Geometry: final body of the model. Coordinates: model frame, mm. Face numbers are marked on the shaded views. A direction names the side the tool comes from. Give positions to 0.01 mm unless a question says otherwise; leave off trailing zeros. Order: outer loops, then holes, each group sorted by start corner. A loop starts at its lowest first (then second) coordinate and runs counter-clockwise, first axis right, second up. Notation, with made-up numbers: (28.5, 59.25) -> (85.5, 59.25) arc R19 cw to (85.5, 85.25) -> close; hole circle Ø11 at (-16, 14.5). An arc over 180 degrees is marked (long way). Answer in a Markdown table with one row per item. Add a question column.
Q1. Set-up query: the marked faces 1 and 2. Return all of +Z, -Z, +X, -X, +Y, -Y with unobstructed straight access to the full face (end or side cutting, diameter ignored); none if empty.
Q2. Line query: line 1 along Z through (x, y) = (533, -532.5); line 2 along Y through (x, z) = (37.5, 875.5); line 3 along X through (y, z) = (-129.5, 848). Output: solid intervals per line, ascending. Write a range as from..to.
Q3. Cut plane A-A on x = 339. Return the cut outline in (y, z).
Q4. Cut plane B-B on y = 458.5. Return the cut outline in (x, z), and give its area (3 significant figures).
from build123d import *

# Parameters (mm, degrees)
F0_W     = 590
F0_H     = 157.407396
F2_W     = 1200
F2_H     = 1200
F3_DEPTH = 842.592604


with BuildPart() as f1:
    # F0 (on Front) → F1 (revolve)
    with BuildSketch(Plane.XZ):
        Polygon((-600, 842.592604), (-600, 0), (0, 0), (0, 842.592604), (-590, 842.592604), align=None)
        with Locations((-295, 921.296302)):
            Rectangle(F0_W, F0_H)
    revolve(axis=Axis((0, 0, 487.345502), (0, 0, -1)))

    # F2 (on face) → F3 (join, through all)
    with BuildSketch(Plane(origin=(0, 0, 0), x_dir=(1, 0, 0), z_dir=(0, 0, -1))):
        Rectangle(F2_W, F2_H)
    extrude(amount=-F3_DEPTH)


solid = f1.part
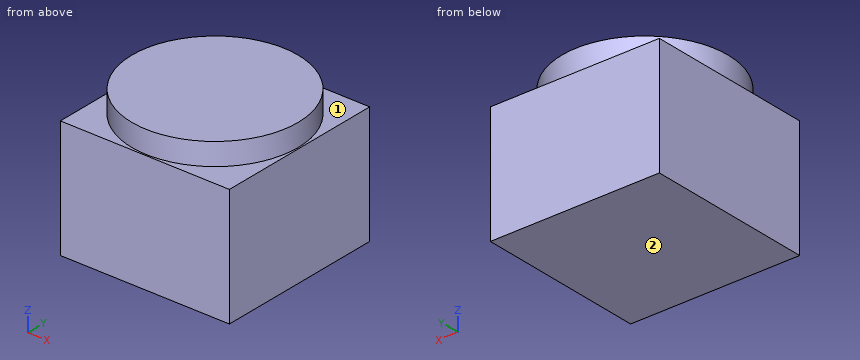
Completed:
| question | item | result |
|---|---|---|
| 1 | face 1 | +Z |
| 1 | face 2 | -Z, +X, -X, +Y, -Y |
| 2 | line 1 | z = 0..842.59 |
| 2 | line 2 | y = -588.81..588.81 |
| 2 | line 3 | x = -575.61..575.61 |
| 3 | outline | (-600, 0) -> (600, 0) -> (600, 842.59) -> (482.89, 842.59) -> (482.89, 1000) -> (-482.89, 1000) -> (-482.89, 842.59) -> (-600, 842.59) -> close |
| 4 | outline | (-600, 0) -> (600, 0) -> (600, 842.59) -> (371.32, 842.59) -> (371.32, 1000) -> (-371.32, 1000) -> (-371.32, 842.59) -> (-600, 842.59) -> close |
| 4 | area | 1,130,000 mm² |
